Here's how the part is built. I have some questions about the finished solid (model axes, mm). Face numbers are marked on the shaded views. A direction names the side the tool comes from. Round coordinates to 2 decimals unless told otherwise and drop trailing zeros. Loops run counter-clockwise (first coordinate to the right, second up) from the corner with the lowest first, then second, coordinate; pieces in that order, holes last. Notation, with made-up numbers: M 11,68.5 L 55,68.5 A16 cw 55,74.5 Z; hole C -6,7 d10. An arc over 180 degrees is marked long. Answer as CSV lines item,"result".
```python
from build123d import *

# Parameters (mm, degrees)
F0_W     = 76.2
F0_H     = 19.05
F1_DEPTH = 152.4


with BuildPart() as f1:
    # F0 (on Front) → F1 (new body)
    with BuildSketch(Plane.XZ):
        with BuildLine():
            Line((46.0375, 60.325), (28.575, 60.325))
            Line((28.575, 60.325), (28.575, 41.275))
            Line((28.575, 41.275), (28.575, -52.705))
            Line((28.575, -52.705), (46.0375, -52.705))
            ThreePointArc((46.0375, -52.705), (47.160032, -52.240032), (47.625, -51.1175))
            Line((47.625, -51.1175), (47.625, 58.7375))
            ThreePointArc((47.625, 58.7375), (47.160032, 59.860032), (46.0375, 60.325))
        make_face()
        with Locations((-9.525, 50.8)):
            Rectangle(F0_W, F0_H)
    extrude(amount=F1_DEPTH)


solid = f1.part
```
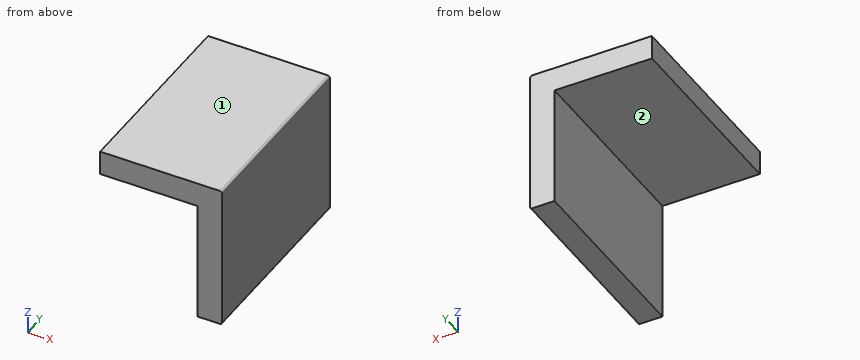
1. For P1, Ø4, axis at y = -63.5, z = -17, coming from the -X side (3 decimals); P2, Ø8, axis at x = -8, y = -114.5, coming from the -Z side (3 decimals), each with a flat end and sliding along its axis, tell me the tip position at first contact or that it passes through.
Evaluation:
P1,"stops at x = 28.575"
P2,"stops at z = 41.275"
2. I want a section at C-C, the plane x = 2.5. Please give me the cut outline in (y, z) (3 decimals), and give its area (3 significant figures).
Evaluation:
outline,"M -152.4,41.275 L 0,41.275 L 0,60.325 L -152.4,60.325 Z"
area,"2,900 mm²"
3. Which directions (+Z, -Z, +X, -X, +Y, -Y) give clear straight access to the entire face, cutting with the end or side of a thin tool? Please do the marked faces 1 and 2.
Evaluation:
face 1,"+Z, +X, -X, +Y, -Y"
face 2,"-Z, -X, +Y, -Y"
4. If I drill on line 1 (Z direction, x = 24, y = -62) (3 decimals); line 2 (X direction, y = -62.5, z = -8.5) (3 decimals), over which ranges is the centre line in solid material (lowest first)? Write a range as [from, to].
Evaluation:
line 1,"z = [41.275, 60.325]"
line 2,"x = [28.575, 47.625]"
5. I want a section at A-A, the plane y = -140.5. Please give me the cut outline in (x, z) (1 decimal).
Evaluation:
outline,"M -47.6,41.3 L 28.6,41.3 L 28.6,-52.7 L 46,-52.7 A1.6 ccw 47.6,-51.1 L 47.6,58.7 A1.6 ccw 46,60.3 L -47.6,60.3 Z"
6. I want a section at B-B, the plane z = -23. Please give me the cut outline in (x, y) (3 decimals), and give its area (3 significant figures).
Evaluation:
outline,"M 28.575,-152.4 L 47.625,-152.4 L 47.625,0 L 28.575,0 Z"
area,"2,900 mm²"
